For this review, take the finished solid that the model builds, in its own axes (mm). Face numbers are marked on the shaded views. A direction names the side the tool comes from. Round coordinates to 2 decimals unless told otherwise and drop trailing zeros. Loops run counter-clockwise (first coordinate to the right, second up) from the corner with the lowest first, then second, coordinate; pieces in that order, holes last.
1. Consider section B-B on z = 0. State how many separate pieces and enclosed holes the cut face has, then the cut area to 3 significant figures.
2. Tool access review of the marked faces 1, 2 and 3: name each direction out of +Z, -Z, +X, -X, +Y, -Y from which nothing blocks a thin tool from reaching the whole face with its end or side.
3. Clearance check with flat-ended pins moving along their axes: pin 1 Ø1.5 at (y, z) = (-26.5, 5) entering from -X; pin 2 Ø5 at (x, z) = (15, -2) entering from -Y; pin 3 Ø2.5 at (x, z) = (-45.085, 0) entering from +Y; pin 4 Ø6.5 at (x, z) = (-61.5, 2) entering from +Y (3 decimals). State where each tip first meets the part, or that it passes through.
4. Consider section D-D on x = 34. State the section outline as (y, z) points.
5. Draft analysis for pull direction X (two halves, no side actions). For the marked faces 4, 5 and 6, state which applies: released by +X, released by -X, zero draft, split by the parting line, or undercut.
6. Consider section A-A on y = -29. State the section outline as (x, z) points.
7. To check wall thickness, follow line 1 along X through (y, z) = (-49.5, 0); line 2 along X through (y, z) = (2.5, 0); line 3 along Z through (x, y) = (63.5, -49.45). State the ranges of each line that lie inside material, in increasing order.
from build123d import *

# Parameters (mm, degrees)
SKETCH1_W           = 114.3
SKETCH1_H           = 12.7
BOSS_EXTRUDE1_DEPTH = 6.35
SKETCH2_W           = 6.35
SKETCH2_H           = 12.7
BOSS_EXTRUDE2_DEPTH = 50.8
SKETCH3_W           = 12.7
SKETCH3_H           = 3.175
BOSS_EXTRUDE3_DEPTH = 12.7
CUT_EXTRUDE1_REACH  = 90.502
SKETCH4_R           = 1.5875
CUT_EXTRUDE2_REACH  = 92.474
SKETCH5_R           = 1.4732


with BuildPart() as part:
    # Sketch1 → Boss-Extrude1 (new body)
    with BuildSketch(Plane(origin=(0, 0, 0), x_dir=(1, 0, 0), z_dir=(0, 1, 0))):
        Rectangle(SKETCH1_W, SKETCH1_H)
    extrude(amount=BOSS_EXTRUDE1_DEPTH)

    # Sketch2 → Boss-Extrude2 (add)
    with BuildSketch(Plane.XZ):
        with Locations((-53.975, 0)):
            Rectangle(SKETCH2_W, SKETCH2_H)
    boss_extrude2 = extrude(amount=BOSS_EXTRUDE2_DEPTH)

    # Sketch3 → Boss-Extrude3 (add)
    with BuildSketch(Plane.ZY.offset(57.15)):
        with Locations((0, -49.2125)):
            Rectangle(SKETCH3_W, SKETCH3_H)
    boss_extrude3 = extrude(amount=BOSS_EXTRUDE3_DEPTH)

    # Mirror1: Boss-Extrude2, Boss-Extrude3 across plane
    add(boss_extrude2.mirror(Plane(origin=(0, 0, 0), x_dir=(0, 0, 1), z_dir=(1, 0, 0))))
    add(boss_extrude3.mirror(Plane(origin=(0, 0, 0), x_dir=(0, 0, 1), z_dir=(1, 0, 0))))

    # Sketch4 → Cut-Extrude1 (cut, up to next)
    with BuildSketch(Plane(origin=(0, -47.625, 0), x_dir=(1, 0, 0), z_dir=(0, 1, 0)), mode=Mode.PRIVATE) as cut_extrude1_sk1:
        with Locations(Location((-63.5, 0, 0), (0, 0, 270))):
            Circle(SKETCH4_R)
    cut_extrude1_tool1 = extrude(cut_extrude1_sk1.sketch, amount=-CUT_EXTRUDE1_REACH, mode=Mode.PRIVATE) & part.part
    cut_extrude1 = cut_extrude1_tool1.solids().sort_by_distance((-63.5, -47.625, 0))[0]
    add(cut_extrude1, mode=Mode.SUBTRACT)

    # Mirror2: Cut-Extrude1 across plane
    add(cut_extrude1.mirror(Plane(origin=(0, 0, 0), x_dir=(0, 0, 1), z_dir=(1, 0, 0))), mode=Mode.SUBTRACT)

    # Sketch5 → Cut-Extrude2 (cut, up to next)
    with BuildSketch(Plane(origin=(0, 6.35, 0), x_dir=(1, 0, 0), z_dir=(0, 1, 0)), mode=Mode.PRIVATE) as cut_extrude2_sk1:
        with Locations(Location((-45.085, 0, 0), (0, 0, 270))):
            Circle(SKETCH5_R)
    cut_extrude2_tool1 = extrude(cut_extrude2_sk1.sketch, amount=-CUT_EXTRUDE2_REACH, mode=Mode.PRIVATE) & part.part
    # Sketch5 → Cut-Extrude2 (cut, up to next)
    with BuildSketch(Plane(origin=(0, 6.35, 0), x_dir=(1, 0, 0), z_dir=(0, 1, 0)), mode=Mode.PRIVATE) as cut_extrude2_sk2:
        with Locations(Location((45.085, 0, 0), (0, 0, 270))):
            Circle(SKETCH5_R)
    cut_extrude2_tool2 = extrude(cut_extrude2_sk2.sketch, amount=-CUT_EXTRUDE2_REACH, mode=Mode.PRIVATE) & part.part
    add(cut_extrude2_tool1.solids().sort_by_distance((-45.085, 6.35, 0))[0], mode=Mode.SUBTRACT)
    add(cut_extrude2_tool2.solids().sort_by_distance((45.085, 6.35, 0))[0], mode=Mode.SUBTRACT)


solid = part.part
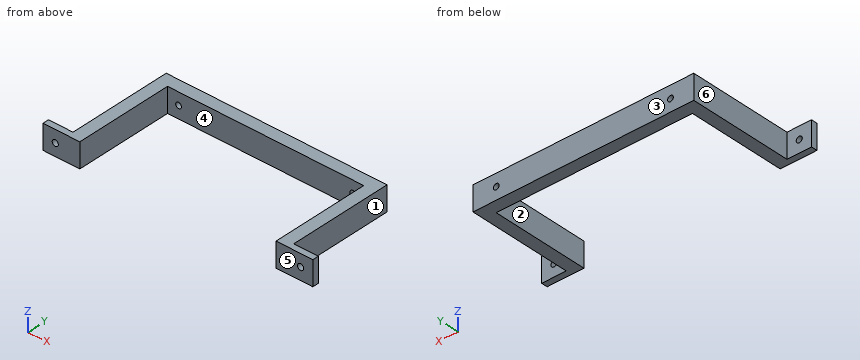
Resolved:
1. separate pieces: 5
1. enclosed holes: 0
1. area: 1,390 mm2
2. face 1: +Z, -Z, +X, +Y
2. face 2: +Z, -Z, -Y
2. face 3: +Z, -Z, +X, -X, +Y
3. pin 1: stops at x = -57.15
3. pin 2: stops at y = 0
3. pin 3: passes through
3. pin 4: stops at y = -47.625
4. outline: (0, -6.35) - (6.35, -6.35) - (6.35, 6.35) - (0, 6.35) - close
5. face 4: undercut
5. face 5: zero draft
5. face 6: released by -X
6. outline: (-57.15, -6.35) - (-50.8, -6.35) - (-50.8, 6.35) - (-57.15, 6.35) - close; (50.8, -6.35) - (57.15, -6.35) - (57.15, 6.35) - (50.8, 6.35) - close
7. line 1: x = -69.85 to -65.09, -61.91 to -50.8, 50.8 to 61.91, 65.09 to 69.85
7. line 2: x = -57.15 to -46.56, -43.61 to 43.61, 46.56 to 57.15
7. line 3: z = -6.35 to -1.59, 1.59 to 6.35
